```python
from build123d import *

# Parameters (mm, degrees)
F1_R     = 34.925
F2_DEPTH = 35.56
F3_R     = 2.54
F4_R     = 28.575
F5_DEPTH = 22.86


with BuildPart() as f2:
    # F1 (on face) → F2 (new body)
    with BuildSketch(Plane.XY):
        Circle(F1_R)
    extrude(amount=F2_DEPTH)

    # F3
    f3_edges = [f2.edges().sort_by_distance(p)[0] for p in [
        (-34.925, 0, 35.56),
    ]]
    fillet(f3_edges, radius=F3_R)

    # F4 (on Top) → F5 (cut)
    with BuildSketch(Plane.XY):
        Circle(F4_R)
    extrude(amount=F5_DEPTH, mode=Mode.SUBTRACT)


solid = f2.part
```
Could you check a few things on this model? Use its own coordinates, in mm. A direction names the side the tool comes from. Coordinates: 2 decimals unless noted, no trailing zeros. Order: outer loops, then holes, each group sorted by start corner. A loop starts at its lowest first (then second) coordinate and runs counter-clockwise, first axis right, second up. Notation, with made-up numbers: M -9.75,35 L 27.25,35 A26 ccw 27.25,57 Z; hole C 38,74 d8. An arc over 180 degrees is marked long. Use a Markdown table: item, result. Add a question column.
Q1. Which directions (+Z, -Z, +X, -X, +Y, -Y) give clear straight access to the entire face, cutting with the end or side of a thin tool? Please do faces 4 (the flat face through (0, 0, 22.86)), 5 (the flat face through (0, 0, 35.56)).
Q2. I want a section at A-A on y = 0. List the corners of the cut face in (x, z) for me (3 decimals).
Q3. I'm going to push flat-ended pins straight in: pin 1 (17 mm diameter, centred on x = -10, y = 7.5, fed in from -Z); pin 2 (4 mm diameter, centred on x = 11, z = 18, fed in from +Y); pin 3 (8 mm diameter, centred on y = 9.5, z = 30.5, fed in from +X). Where does each tip first touch, or does it pass through?
Q4. We'd pull the mould along Y, two halves only. Please class faces 1 (the cylindrical face through (-27.715, -21.251, 16.279)), 2 (the flat face through (-29, 0, 0)), 3 (the cylindrical face through (-28.547, 1.256, 11.27)): pulls with the +Y half, pulls with the -Y half, needs draft (parallel to the pull), parting line crosses it, or undercut.
Q5. I want a section at D-D on z = 30. List the corners of the cut face in (x, y) for me (3 decimals), then the cut area to 3 significant figures.
Q6. If I drill on L1, parallel to Y at x = 0, z = 13.5 (3 decimals); L2, parallel to Y at x = -24, z = 12.5; L3, parallel to Z at x = -22.5, y = -14, over which ranges is the centre line in solid material (lowest first)?
Q7. I want a section at C-C on z = 15. List the corners of the cut face in (x, y) for me (3 decimals), then the cut area to 3 significant figures.
Checked values:
| question | item | result |
|---|---|---|
| 1 | face 4 | -Z |
| 1 | face 5 | +Z, +X, -X, +Y, -Y |
| 2 | outline | M -34.925,0 L -28.575,0 L -28.575,22.86 L 28.575,22.86 L 28.575,0 L 34.925,0 L 34.925,33.02 A2.54 ccw 32.385,35.56 L -32.385,35.56 A2.54 ccw -34.925,33.02 Z |
| 3 | pin 1 | z = 22.86 |
| 3 | pin 2 | y = 33.75 |
| 3 | pin 3 | x = 34.49 |
| 4 | face 1 | parting line crosses it |
| 4 | face 2 | needs draft |
| 4 | face 3 | undercut |
| 5 | outline | C 0,0 d69.85 |
| 5 | area | 3,830 mm² |
| 6 | L1 | -34.925 to -28.575, 28.575 to 34.925 |
| 6 | L2 | -25.37 to -15.51, 15.51 to 25.37 |
| 6 | L3 | 22.86 to 35.56 |
| 7 | outline | C 0,0 d69.85; hole C 0,0 d57.15 |
| 7 | area | 1,270 mm² |
